Verification items for this drawing (mm, ordinates from the low corner). A direction names the side the tool comes from. Round coordinates to 2 decimals unless told otherwise and drop trailing zeros. Write each loop counter-clockwise with the first axis right and the second up, starting at its lowest first coordinate (ties: lowest second). Pieces come first, ordered by that corner, then holes. Notation, with made-up numbers: M -15.75,-12 L 29.25,-12 A23 cw 29.25,6 Z; hole C 77.25,-24.75 d3. An arc over 180 degrees is marked long. One line per question, with ' | ' between items. Start each with the question number.
Q1. Gauge pin test, flat ends, axial feed: pin 1 (6 mm diameter, centred on y = 35, z = 83.5, fed in from +X); pin 2 (22 mm diameter, centred on x = 60.5, y = 27.5, fed in from -Z); pin 3 (8.5 mm diameter, centred on x = 60.5, y = 33, fed in from +Z). Record the tip position at first contact, or that the pin passes through.
Q2. Cross-section at D-D (y = 32.5). Record the boundary of the cut face in (x, z), then the cut area to 3 significant figures.
Q3. Cross-section at A-A (z = 78). State how many separate pieces and enclosed holes the cut face has, then the cut area to 3 significant figures.
Q4. Cross-section at C-C (y = 15.5). Record the boundary of the cut face in (x, z), then the cut area to 3 significant figures.
Q5. Release check for a two-part mould opening along Z. For the marked faces 1, 2 and 3 record: released by +Z, released by -Z, zero draft, split by the parting line, or undercut.
Q6. Tool access check on the marked faces 4, 5, 6 and 7. Record the directions out of +Z, -Z, +X, -X, +Y, -Y that give a thin tool (end or side, any length) a straight path to the whole face; none if there is none.
Q7. Thickness scan on line 1 along Z through (x, y) = (102.5, 39); line 2 along Y through (x, z) = (55, 15.75); line 3 along Y through (x, z) = (87, 63). Record the ranges inside material, lowest first. Write a range as from..to.
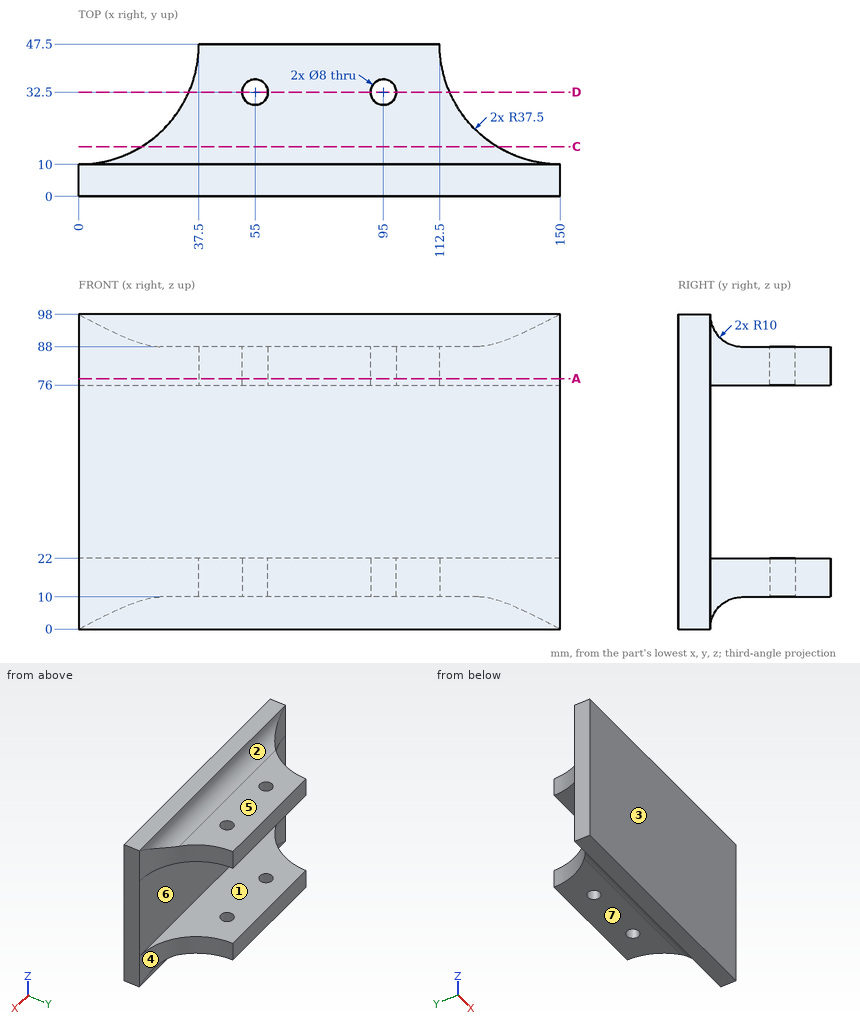
Determined:
1) pin 1: stops at x = 115.85 | pin 2: stops at z = 9.37 | pin 3: stops at z = 88
2) outline: M 34.37,10 L 51,10 L 51,22 L 34.37,22 Z; M 34.37,76 L 51,76 L 51,88 L 34.37,88 Z; M 59,10 L 91,10 L 91,22 L 59,22 Z; M 59,76 L 91,76 L 91,88 L 59,88 Z; M 99,10 L 115.63,10 L 115.63,22 L 99,22 Z; M 99,76 L 115.63,76 L 115.63,88 L 99,88 Z | area: 1,570 mm²
3) separate pieces: 1 | enclosed holes: 2 | area: 4,820 mm²
4) outline: M 19.55,8.93 L 130.45,8.93 L 130.45,22 L 19.55,22 Z; M 19.55,76 L 130.45,76 L 130.45,89.07 L 19.55,89.07 Z | area: 2,900 mm²
5) face 1: undercut | face 2: released by +Z | face 3: zero draft
6) face 4: +Z, -Z, +X, +Y | face 5: +Z, +X, -X, +Y | face 6: +X, -X, +Y | face 7: -Z, +X, -X, +Y
7) line 1: z = 10..22, 76..88 | line 2: y = 0..28.5, 36.5..47.5 | line 3: y = 0..10
